Check sheet for the drawn part. Datum: minimum x, y, z corner. Units: mm. Give positions to 0.01 mm unless a question says otherwise; leave off trailing zeros. Write each loop counter-clockwise with the first axis right and the second up, starting at its lowest first coordinate (ties: lowest second). Pieces come first, ordered by that corner, then holes. Notation, with made-up numbers: (-37, -1.5) - (-32, -1.5) arc R17 cw to (-32, 21.5) - close; hole circle Ø6 at (43.25, 46.5). An arc over 180 degrees is marked (long way). Use a Markdown table: item, result.
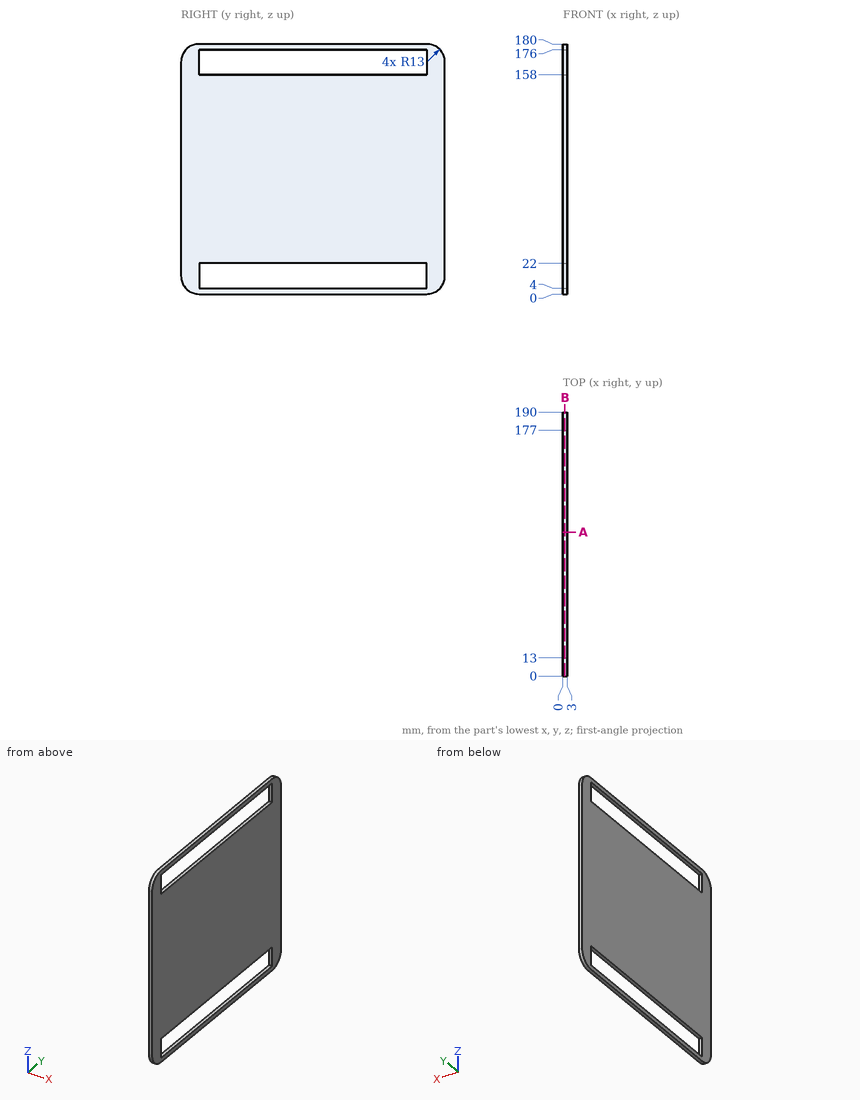
1) Material ranges on L1, parallel to Z at x = 2.7, y = 118.5; L2, parallel to Y at x = 1.35, z = 12, recorded low to high. Write a range as from..to.
Working result:
| item | result |
|---|---|
| L1 | z = 0..4, 22..158, 176..180 |
| L2 | y = 0.04..13, 177..189.96 |
2) Section check B-B on x = 1.35. Record the boundary of the cut face in (y, z).
Working result:
| item | result |
|---|---|
| outline | (0, 13) arc R13 ccw to (13, 0) - (177, 0) arc R13 ccw to (190, 13) - (190, 167) arc R13 ccw to (177, 180) - (13, 180) arc R13 ccw to (0, 167) - close; hole (13, 4) - (177, 4) - (177, 22) - (13, 22) - close; hole (13, 158) - (177, 158) - (177, 176) - (13, 176) - close |
3) Depth check by flat-ended pin: P1, Ø0.9, axis at x = 1.5, z = 168.5, coming from the +Y side; P2, Ø1.5, axis at x = 1, z = 11, coming from the -Y side. Enter the tip coordinate at first touch or a pass-through.
Working result:
| item | result |
|---|---|
| P1 | stops at y = 189.96 |
| P2 | stops at y = 0.06 |
4) Section check A-A on y = 103.5. Record the boundary of the cut face in (x, z).
Working result:
| item | result |
|---|---|
| outline | (0, 0) - (3, 0) - (3, 4) - (0, 4) - close; (0, 22) - (3, 22) - (3, 158) - (0, 158) - close; (0, 176) - (3, 176) - (3, 180) - (0, 180) - close |
